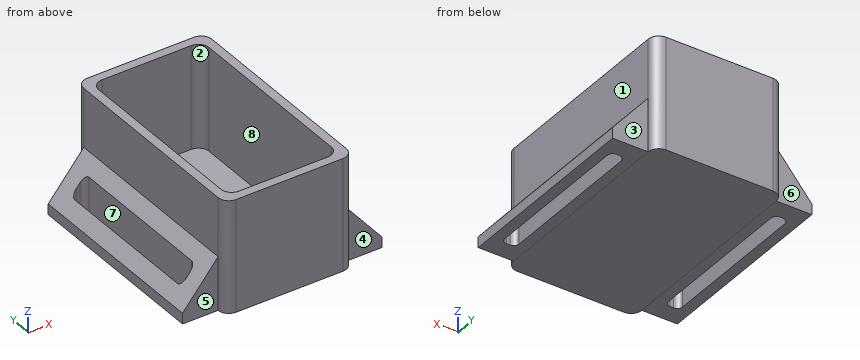
from build123d import *

# Parameters (mm, degrees)
SHELL_DEPTH         = 29
BOTTOM_START        = 2.5
BOTTOM_COVER_DEPTH  = 2.5
BOSS_EXTRUDE4_DEPTH = 55
CUT_EXTRUDE1_DEPTH  = 64


with BuildPart() as part:
    # Sketch1 → Shell (new body)
    with BuildSketch(Plane.XY):
        with BuildLine():
            Line((-14.99046496, 38.43538022), (15.00953504, 38.43538022))
            ThreePointArc((15.00953504, 38.43538022), (17.130855384, 37.556700564), (18.00953504, 35.43538022))
            Line((18.00953504, 35.43538022), (18.00953504, -19.56461978))
            ThreePointArc((18.00953504, -19.56461978), (17.130855384, -21.685940124), (15.00953504, -22.56461978))
            Line((15.00953504, -22.56461978), (-14.99046496, -22.56461978))
            ThreePointArc((-14.99046496, -22.56461978), (-17.111785303, -21.685940124), (-17.99046496, -19.56461978))
            Line((-17.99046496, -19.56461978), (-17.99046496, 35.43538022))
            ThreePointArc((-17.99046496, 35.43538022), (-17.111785303, 37.556700564), (-14.99046496, 38.43538022))
        make_face()
        with BuildLine():
            Line((-12.49046496, 35.93538022), (12.50953504, 35.93538022))
            ThreePointArc((12.50953504, 35.93538022), (14.630855384, 35.056700564), (15.50953504, 32.93538022))
            Line((15.50953504, 32.93538022), (15.50953504, -17.06461978))
            ThreePointArc((15.50953504, -17.06461978), (14.630855384, -19.185940124), (12.50953504, -20.06461978))
            Line((12.50953504, -20.06461978), (-12.49046496, -20.06461978))
            ThreePointArc((-12.49046496, -20.06461978), (-14.611785303, -19.185940124), (-15.49046496, -17.06461978))
            Line((-15.49046496, -17.06461978), (-15.49046496, 32.93538022))
            ThreePointArc((-15.49046496, 32.93538022), (-14.611785303, 35.056700564), (-12.49046496, 35.93538022))
        make_face(mode=Mode.SUBTRACT)
    extrude(amount=SHELL_DEPTH)

    # Sketch3 → Bottom cover (add)
    with BuildSketch(Plane(origin=(0, 0, 0), x_dir=(-1, 0, 0), z_dir=(0, 0, -1)).offset(BOTTOM_START)):
        with BuildLine():
            Line((-15.00953504, 38.43538022), (14.99046496, 38.43538022))
            ThreePointArc((14.99046496, 38.43538022), (17.111785303, 37.556700564), (17.99046496, 35.43538022))
            Line((17.99046496, 35.43538022), (17.99046496, -19.56461978))
            ThreePointArc((17.99046496, -19.56461978), (17.111785303, -21.685940124), (14.99046496, -22.56461978))
            Line((14.99046496, -22.56461978), (-15.00953504, -22.56461978))
            ThreePointArc((-15.00953504, -22.56461978), (-17.130855384, -21.685940124), (-18.00953504, -19.56461978))
            Line((-18.00953504, -19.56461978), (-18.00953504, 35.43538022))
            ThreePointArc((-18.00953504, 35.43538022), (-17.130855384, 37.556700564), (-15.00953504, 38.43538022))
        make_face()
    extrude(amount=-BOTTOM_COVER_DEPTH)


with BuildPart() as boss_extrude4_tool:
    # 3DSketch1 → Boss-Extrude4 (new body)
    with BuildSketch(Plane(origin=(18.009536245, 35.43538022, -2.500000038), x_dir=(-0.99788010602318, 0, 0.06507913646605183), z_dir=(0, 1, 0))):
        Polygon((0, 0), (-9.97880106, 0.650791365), (-9.783563651, 3.644431683), (0.976187047, 14.96820159), align=None)
        Polygon((35.923685021, -2.342848953), (45.902486082, -2.993640318), (46.097723491, 0), (36.899872068, 12.625352637), align=None)
    extrude(amount=-BOSS_EXTRUDE4_DEPTH)


with BuildPart() as part_1:
    add(part.part)


with BuildPart() as part_2:
    # Boss-Extrude4: joined with boss_extrude4_tool
    add(part_1.part.fuse(boss_extrude4_tool.part, tol=0.00001))

    # Sketch9 → Cut-Extrude1 (cut)
    with BuildSketch(Plane(origin=(0, 0, -2.5), x_dir=(-1, 0, 0), z_dir=(0, 0, -1))):
        with BuildLine():
            Line((-23.50953504, -14.56461978), (-22.50953504, -14.56461978))
            ThreePointArc((-22.50953504, -14.56461978), (-21.448874869, -14.125279952), (-21.00953504, -13.06461978))
            Line((-21.00953504, -13.06461978), (-21.00953504, 28.93538022))
            ThreePointArc((-21.00953504, 28.93538022), (-21.448874869, 29.996040392), (-22.50953504, 30.43538022))
            Line((-22.50953504, 30.43538022), (-23.50953504, 30.43538022))
            ThreePointArc((-23.50953504, 30.43538022), (-24.570195212, 29.996040392), (-25.00953504, 28.93538022))
            Line((-25.00953504, 28.93538022), (-25.00953504, -13.06461978))
            ThreePointArc((-25.00953504, -13.06461978), (-24.570195212, -14.125279952), (-23.50953504, -14.56461978))
        make_face()
        with BuildLine():
            Line((22.49046496, 30.43538022), (23.49046496, 30.43538022))
            ThreePointArc((23.49046496, 30.43538022), (24.551125131, 29.996040392), (24.99046496, 28.93538022))
            Line((24.99046496, 28.93538022), (24.99046496, -13.06461978))
            ThreePointArc((24.99046496, -13.06461978), (24.551125131, -14.125279952), (23.49046496, -14.56461978))
            Line((23.49046496, -14.56461978), (22.49046496, -14.56461978))
            ThreePointArc((22.49046496, -14.56461978), (21.429804788, -14.125279952), (20.99046496, -13.06461978))
            Line((20.99046496, -13.06461978), (20.99046496, 28.93538022))
            ThreePointArc((20.99046496, 28.93538022), (21.429804788, 29.996040392), (22.49046496, 30.43538022))
        make_face()
    extrude(amount=-CUT_EXTRUDE1_DEPTH, mode=Mode.SUBTRACT)


solid = part_2.part
The model under review builds one solid part; all positions refer to its coordinate system, in mm. Face numbers are marked on the shaded views. A direction names the side the tool comes from. Give positions to 0.01 mm unless a question says otherwise; leave off trailing zeros. Loops run counter-clockwise (first coordinate to the right, second up) from the corner with the lowest first, then second, coordinate; pieces in that order, holes last. Notation, with made-up numbers: (-18, -2) -> (7, -2) arc R21 ccw to (7, 16) -> close; hole circle Ø9 at (-3.75, 43.25). An arc over 180 degrees is marked (long way). Answer as a JSON object with one key per item and string values. Group by question number.
Q1. Draft analysis for pull direction X (two halves, no side actions). For the marked faces 1, 2 and 3, state which applies: pulls with the +X half, pulls with the -X half, needs draft (parallel to the pull), parting line crosses it, or undercut.
Q2. Tool access review of the marked faces 4, 5, 6, 7 and 8: name each direction out of +Z, -Z, +X, -X, +Y, -Y from which nothing blocks a thin tool from reaching the whole face with its end or side.
Q3. Take a section at C-C (x = -8). Write out the cut boundary in (y, z).
Q4. Take a section at D-D (z = 8). Write out the cut boundary in (x, y).
Q5. Insertion check: pin 1 (8 mm diameter, centred on y = -8.5, z = 25.5, fed in from +X); pin 2 (6 mm diameter, centred on y = 11.5, z = 9, fed in from +X); pin 3 (8 mm diameter, centred on x = -23, z = 1.5, fed in from -Y). Each pin has a flat end and moves straight along its axis. Give the tip position at first contact, or say it passes through.
Q6. Take a section at B-B (y = 22.5). Write out the cut boundary in (x, z).
Q7. Wall thickness on line 1 along Y through (x, z) = (-5.5, 18); line 2 along X through (y, z) = (11.5, 1.5); line 3 along X through (y, z) = (31, 14.5): over which ranges is each line inside the solid? List them lowest first.
Q8. Take a section at A-A (z = 24.5). Write out the cut boundary in (x, y), plus the area to 3 significant figures.
Answer below:
{
 "1": {"face 1": "pulls with the +X half", "face 2": "undercut", "face 3": "needs draft"},
 "2": {"face 4": "+Z, -Z, +X, -Y", "face 5": "+Z, -Z, -X, -Y", "face 6": "+Z, -Z, -X, +Y", "face 7": "+Z, -Z", "face 8": "+Z"},
 "3": {"outline": "(-22.56, -2.5) -> (38.44, -2.5) -> (38.44, 29) -> (35.94, 29) -> (35.94, 0) -> (-20.06, 0) -> (-20.06, 29) -> (-22.56, 29) -> close"},
 "4": {"outline": "(-21.74, -19.56) -> (-17.99, -19.56) arc R3 ccw to (-14.99, -22.56) -> (15.01, -22.56) arc R3 ccw to (18.01, -19.56) -> (21.76, -19.56) -> (21.76, -14.36) arc R1.5 cw to (21.01, -13.06) -> (21.01, 28.94) arc R1.5 cw to (21.76, 30.23) -> (21.76, 35.44) -> (18.01, 35.44) arc R3 ccw to (15.01, 38.44) -> (-14.99, 38.44) arc R3 ccw to (-17.99, 35.44) -> (-21.74, 35.44) -> (-21.74, 30.23) arc R1.5 cw to (-20.99, 28.94) -> (-20.99, -13.06) arc R1.5 cw to (-21.74, -14.36) -> close; hole (-15.49, -17.06) arc R3 ccw to (-12.49, -20.06) -> (12.51, -20.06) arc R3 ccw to (15.51, -17.06) -> (15.51, 32.94) arc R3 ccw to (12.51, 35.94) -> (-12.49, 35.94) arc R3 ccw to (-15.49, 32.94) -> close"},
 "5": {"pin 1": "stops at x = 18.01", "pin 2": "stops at x = 21.01", "pin 3": "stops at y = -19.56"},
 "6": {"outline": "(-27.99, -2.5) -> (-24.99, -2.5) -> (-24.99, 4.1) -> (-27.99, 0.5) -> close; (-20.99, -2.5) -> (21.01, -2.5) -> (21.01, 8.9) -> (18.01, 12.5) -> (18.01, 29) -> (15.51, 29) -> (15.51, 0) -> (-15.49, 0) -> (-15.49, 29) -> (-17.99, 29) -> (-17.99, 12.5) -> (-20.99, 8.9) -> close; (25.01, -2.5) -> (28.01, -2.5) -> (28.01, 0.5) -> (25.01, 4.1) -> close"},
 "7": {"line 1": "y = -22.56 to -20.06, 35.94 to 38.44", "line 2": "x = -27.16 to -24.99, -20.99 to -15.49, 15.51 to 21.01, 25.01 to 27.18", "line 3": "x = -17.99 to -15.49, 15.51 to 18.01"},
 "8": {"outline": "(-17.99, -19.56) arc R3 ccw to (-14.99, -22.56) -> (15.01, -22.56) arc R3 ccw to (18.01, -19.56) -> (18.01, 35.44) arc R3 ccw to (15.01, 38.44) -> (-14.99, 38.44) arc R3 ccw to (-17.99, 35.44) -> close; hole (-15.49, -17.06) arc R3 ccw to (-12.49, -20.06) -> (12.51, -20.06) arc R3 ccw to (15.51, -17.06) -> (15.51, 32.94) arc R3 ccw to (12.51, 35.94) -> (-12.49, 35.94) arc R3 ccw to (-15.49, 32.94) -> close", "area": "460 mm2"}
}
